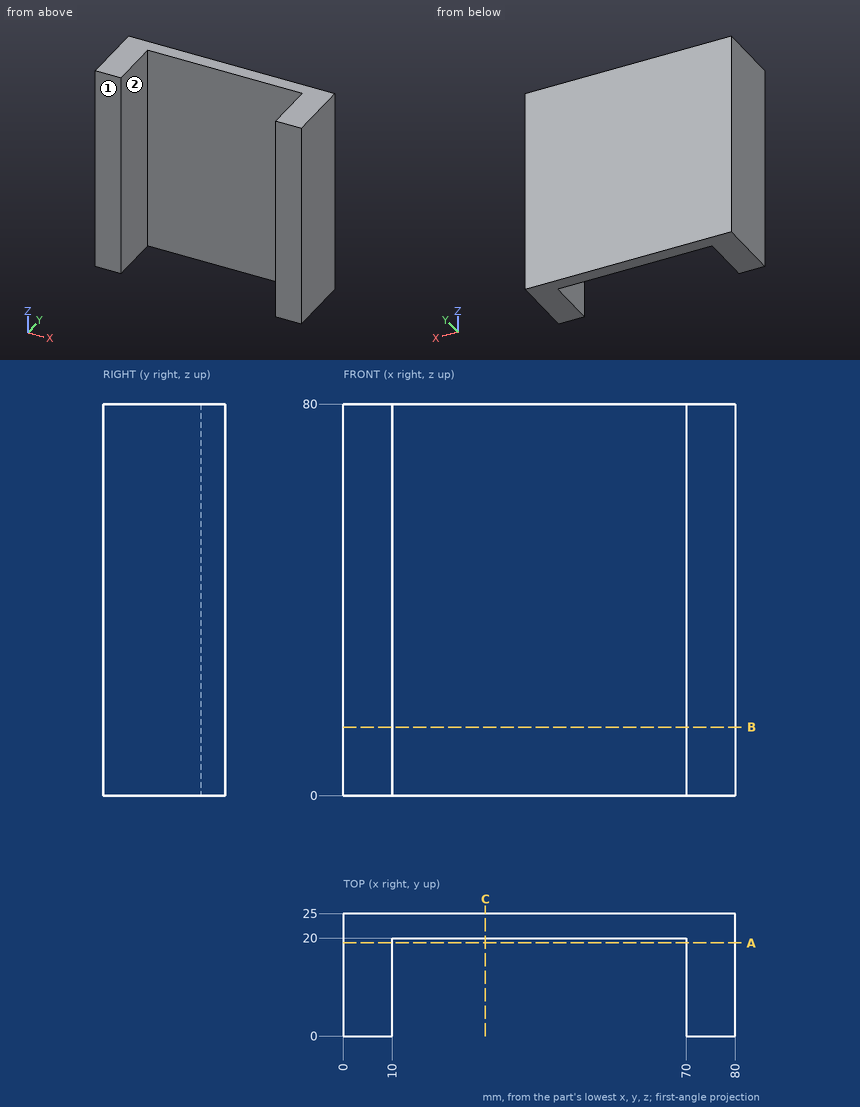
For this review, use the dimensioned drawing (mm, ordinates from the lowest corner) and the shaded views. A direction names the side the tool comes from. Coordinates: 2 decimals unless noted, no trailing zeros. Loops run counter-clockwise (first coordinate to the right, second up) from the corner with the lowest first, then second, coordinate; pieces in that order, holes last.
1. Add section B-B, the plane z = 14. Give the boundary of the cut face in (x, y), then the cut area to 3 significant figures.
2. For the marked faces 1 and 2, list the 3-axis set-ups (+Z, -Z, +X, -X, +Y, -Y) from which the entire face can be reached by the end or side of a thin tool; tool diameter is ignored.
3. Add section C-C, the plane x = 29. Give the boundary of the cut face in (y, z), then the cut area to 3 significant figures.
4. Add section A-A, the plane y = 19. Give the boundary of the cut face in (x, z).
5. For line 1 (X direction, y = 16, z = 22.5); line 2 (Y direction, x = 63.5, z = 4), list the stretches that pass through material, from the lowest coordinate up.
Result:
1. outline: (0, 0) - (10, 0) - (10, 20) - (70, 20) - (70, 0) - (80, 0) - (80, 25) - (0, 25) - close
1. area: 800 mm2
2. face 1: +Z, -Z, +X, -X, -Y
2. face 2: +Z, -Z, -Y
3. outline: (20, 0) - (25, 0) - (25, 80) - (20, 80) - close
3. area: 400 mm2
4. outline: (0, 0) - (10, 0) - (10, 80) - (0, 80) - close; (70, 0) - (80, 0) - (80, 80) - (70, 80) - close
5. line 1: x = 0 to 10, 70 to 80
5. line 2: y = 20 to 25
